Check sheet for the modelled part. Datum: model origin and axes. Units: mm. A direction names the side the tool comes from. Give positions to 0.01 mm unless a question says otherwise; leave off trailing zeros. Loops run counter-clockwise (first coordinate to the right, second up) from the corner with the lowest first, then second, coordinate; pieces in that order, holes last. Notation, with made-up numbers: (-33, 23) - (21, 23) arc R11 ccw to (21, 36) - close; hole circle Ø3 at (-22, 36). An arc over 180 degrees is marked (long way). Answer in a Markdown table with one row per item. Add a question column.
(1) Sectioned sample at B-B on y = -35. Enter the section's corners in (x, z).
(2) Draft check along X on faces 1 (the face through (47.07, -114, 18)), 2 (the face through (47.07, -38, -44)), 3 (the face through (-54.53, -38, -45)), 4 (the face through (72, -38, -70.066)). Enter one of: released by +X, released by -X, zero draft, split by the parting line, or undercut.
(3) Thickness scan on L1, parallel to X at y = -73, z = -55; L2, parallel to X at y = -143.5, z = 22; L3, parallel to Y at x = 76, z = -4. Record the ranges inside material, lowest first.
(4) Sectioned sample at C-C on z = 18. Enter the section's corners in (x, y), then the cut area to 3 significant figures.
(5) Set-up check for faces 5 (the face through (-4, -75, -19.266)), 6 (the face through (-80, -76.2, -6)), 7 (the face through (-105.33, -38, -6)), 8 (the face through (72, -76.2, -6)): record each of +Z, -Z, +X, -X, +Y, -Y from which the full face is reachable in a straight line by a thin tool's end or side.
(6) Sectioned sample at A-A on z = -56. Enter the section's corners in (x, y), then the cut area to 3 significant figures.
(7) Sectioned sample at D-D on x = 62. Enter the section's corners in (y, z).
(8) Go/stop test with flat-tipped pins: P1, Ø4, axis at x = -33, y = -49, coming from the -Z side; P2, Ø3, axis at x = -58, z = -5.5, coming from the -Y side. Record where each tip stops, or that it passes through.
from build123d import *

# Parameters (mm, degrees)
F0_W     = 101.6
F0_H     = 76.2
F1_DEPTH = 76.2
F2_W     = 101.6
F2_H     = 76.2
F3_DEPTH = 76.2


with BuildPart() as f1:
    # F0 (on Front) → F1 (new body)
    with BuildSketch(Plane.XZ):
        with Locations((-3.729625, 18.833704)):
            Rectangle(F0_W, F0_H)
        Polygon((-54.529625, -19.266296), (-54.529625, 56.933704), (-105.329625, 56.933704), (-105.329625, -70.066296), (-54.529625, -70.066296), align=None)
        Polygon((97.870375, 56.933704), (47.070375, 56.933704), (47.070375, -19.266296), (47.070375, -70.066296), (97.870375, -70.066296), align=None)
    extrude(amount=F1_DEPTH)

    # F2 (on face) → F3 (join)
    with BuildSketch(Plane.XZ.offset(76.2)):
        with Locations((-3.729625, 18.833704)):
            Rectangle(F2_W, F2_H)
    extrude(amount=F3_DEPTH)


solid = f1.part
Reply:
| question | item | result |
|---|---|---|
| 1 | outline | (-105.33, -70.07) - (-54.53, -70.07) - (-54.53, -19.27) - (47.07, -19.27) - (47.07, -70.07) - (97.87, -70.07) - (97.87, 56.93) - (-105.33, 56.93) - close |
| 2 | face 1 | released by +X |
| 2 | face 2 | undercut |
| 2 | face 3 | undercut |
| 2 | face 4 | zero draft |
| 3 | L1 | -105.33 to -54.53, 47.07 to 97.87 |
| 3 | L2 | -54.53 to 47.07 |
| 3 | L3 | -76.2 to 0 |
| 4 | outline | (-105.33, -76.2) - (-54.53, -76.2) - (-54.53, -152.4) - (47.07, -152.4) - (47.07, -76.2) - (97.87, -76.2) - (97.87, 0) - (-105.33, 0) - close |
| 4 | area | 23,200 mm^2 |
| 5 | face 5 | -Z, +Y, -Y |
| 5 | face 6 | +Z, -Z, -X, -Y |
| 5 | face 7 | +Z, -Z, -X, +Y, -Y |
| 5 | face 8 | +Z, -Z, +X, -Y |
| 6 | outline | (-105.33, -76.2) - (-54.53, -76.2) - (-54.53, 0) - (-105.33, 0) - close; (47.07, -76.2) - (97.87, -76.2) - (97.87, 0) - (47.07, 0) - close |
| 6 | area | 7,740 mm^2 |
| 7 | outline | (-76.2, -70.07) - (0, -70.07) - (0, 56.93) - (-76.2, 56.93) - close |
| 8 | P1 | z = -19.27 |
| 8 | P2 | y = -76.2 |
